Source: three-view drawing plus pictorial views. Frame: mm from the lowest corner of the part. A direction names the side the tool comes from. Round coordinates to 2 decimals unless told otherwise and drop trailing zeros. Order: outer loops, then holes, each group sorted by start corner. A loop starts at its lowest first (then second) coordinate and runs counter-clockwise, first axis right, second up. Notation, with made-up numbers: (13, 15.5) -> (31, 15.5) arc R16 cw to (31, 43.5) -> close; hole circle Ø7 at (26, 69). An arc over 180 degrees is marked (long way). Use a Markdown table: item, result.
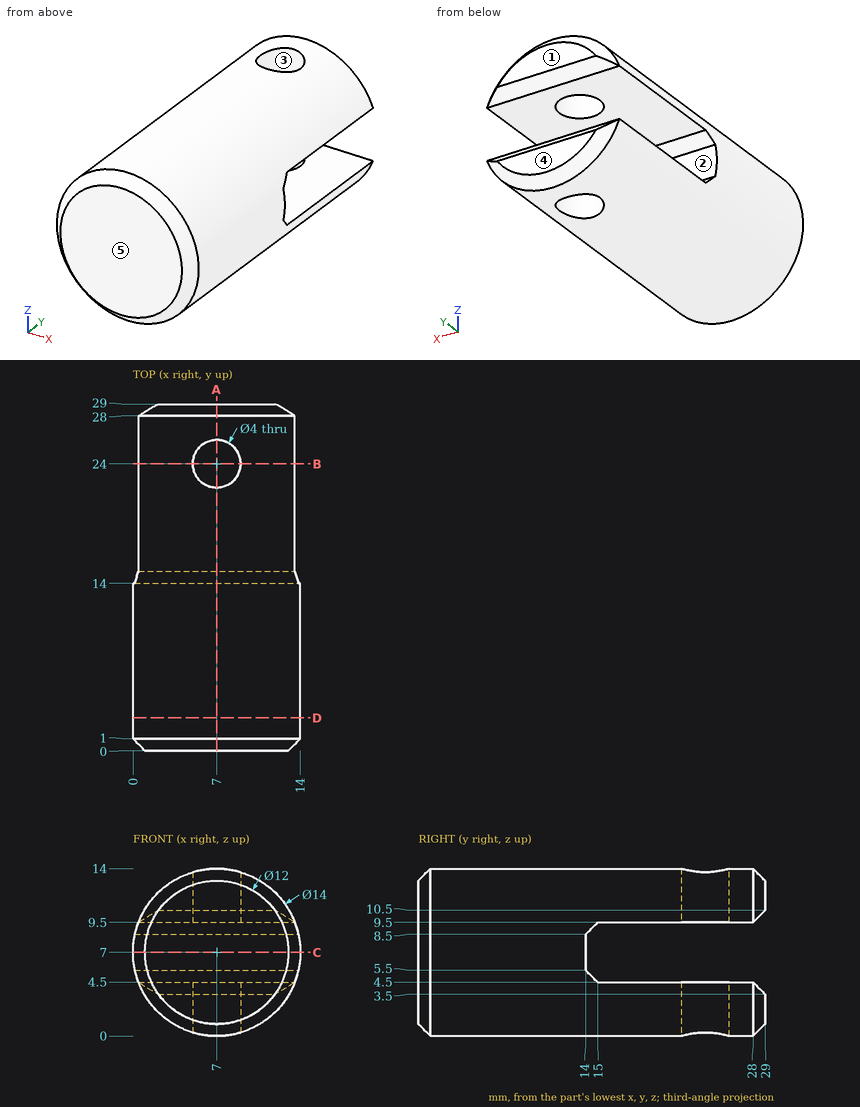
1) Cut plane A-A on x = 7. Return loops of the section in (y, z).
Results found:
| item | result |
|---|---|
| outline | (0, 1) -> (1, 0) -> (22, 0) -> (22, 4.5) -> (15, 4.5) -> (14, 5.5) -> (14, 8.5) -> (15, 9.5) -> (22, 9.5) -> (22, 14) -> (1, 14) -> (0, 13) -> close; (26, 0) -> (28, 0) -> (29, 1) -> (29, 3.5) -> (28, 4.5) -> (26, 4.5) -> close; (26, 9.5) -> (28, 9.5) -> (29, 10.5) -> (29, 13) -> (28, 14) -> (26, 14) -> close |
2) Pin query (flat end, axial travel): pin 1 Ø1.5 at (x, z) = (6.5, 7) entering from +Y; pin 2 Ø1.5 at (y, z) = (24, 6.5) entering from +X; pin 3 Ø1.5 at (x, y) = (5.5, 26) entering from +Z; pin 4 Ø3 at (x, y) = (3, 7) entering from +Z. Return the tip coordinate at first contact, or that it passes through.
Results found:
| item | result |
|---|---|
| pin 1 | stops at y = 14 |
| pin 2 | passes through |
| pin 3 | stops at z = 13.96 |
| pin 4 | stops at z = 13.54 |
3) Set-up query: the marked faces 1 and 2. Return all of +Z, -Z, +X, -X, +Y, -Y with unobstructed straight access to the full face (end or side cutting, diameter ignored); none if empty.
Results found:
| item | result |
|---|---|
| face 1 | +Z, -Z, +X, -X, +Y |
| face 2 | +X, -X, +Y |
4) Cut plane C-C on z = 7. Return loops of the section in (x, y), and give its area (3 significant figures).
Results found:
| item | result |
|---|---|
| outline | (0, 1) -> (1, 0) -> (13, 0) -> (14, 1) -> (14, 14) -> (0, 14) -> close |
| area | 195 mm² |
5) Line query: L1, parallel to X at y = 24, z = 11.15; L2, parallel to X at y = 24, z = 11.4; L3, parallel to Y at x = 6, z = 12. Output: solid intervals per line, ascending. Write a range as [from, to].
Results found:
| item | result |
|---|---|
| L1 | x = [1.36, 5], [9, 12.64] |
| L2 | x = [1.56, 5], [9, 12.44] |
| L3 | y = [0, 22.27], [25.73, 29] |
6) Cut plane B-B on y = 24. Return loops of the section in (x, z).
Results found:
| item | result |
|---|---|
| outline | (0.46, 4.5) arc R7 ccw to (5, 0.29) -> (5, 4.5) -> close; (0.46, 9.5) -> (5, 9.5) -> (5, 13.71) arc R7 ccw to start; (9, 0.29) arc R7 ccw to (13.54, 4.5) -> (9, 4.5) -> close; (9, 9.5) -> (13.54, 9.5) arc R7 ccw to (9, 13.71) -> close |
7) Pull-direction query (Y, two-part tool) for the marked faces 3, 4 and 5; classes: +Y half, -Y half, draft (parallel to the pull), parting line (faces both ways), or undercut.
Results found:
| item | result |
|---|---|
| face 3 | undercut |
| face 4 | +Y half |
| face 5 | -Y half |
8) Cut plane D-D on y = 2.75. Return loops of the section in (x, z).
Results found:
| item | result |
|---|---|
| outline | circle Ø14 at (7, 7) |
